Work out the finished part from the listing and answer in its coordinate system (mm). A direction names the side the tool comes from. Give positions to 0.01 mm unless a question says otherwise; leave off trailing zeros. Loops run counter-clockwise (first coordinate to the right, second up) from the corner with the lowest first, then second, coordinate; pieces in that order, holes last. Notation, with made-up numbers: (-36.75, 50) - (3.25, 50) arc R20 ccw to (3.25, 66) - close; hole circle Ø3 at (45, 31). An arc over 180 degrees is marked (long way). One line per item, written item: value.
Autodesk Inventor part; units mm, degrees
ref_plane "YZ Plane" through (0, 0, 0) normal (1, 0, 0) x (0, 1, 0)
ref_plane "XZ Plane" through (0, 0, 0) normal (0, 1, 0) x (-1, 0, 0)
ref_plane "XY Plane" through (0, 0, 0) normal (0, 0, 1) x (1, 0, 0)
sketch "Sketch1" plane through (0, 0, 0) normal (0, 1, 0) x (-1, 0, 0)
  line L0 (0, 0) -> (2.032, 0) construction
  line L1 (0, 0) -> (-2.032, 0) construction
  line L2 (-4.318, 0) -> (-4.318, 3.81)
  line L3 (-4.318, 3.81) -> (5.842, 3.81)
  line L4 (-2.032, 0) -> (-2.032, 1.651)
  line L5 (-2.032, 1.651) -> (2.032, 1.651)
  line L6 (2.032, -46.228) -> (-2.032, -46.228)
  line L7 (-2.032, -46.228) -> (-2.032, -44.577)
  line L8 (-4.318, -44.577) -> (-4.318, -48.387)
  line L9 (-4.318, -48.387) -> (5.842, -48.387)
  line L10 (2.032, 1.651) -> (2.032, -16.5735)
  line L11 (2.032, -16.5735) -> (4.572, -16.5735)
  line L12 (4.572, -16.5735) -> (4.572, -28.0035)
  line L13 (4.572, -28.0035) -> (2.032, -28.0035)
  line L14 (2.032, -28.0035) -> (2.032, -46.228)
  line L15 (5.842, 3.81) -> (5.842, -48.387)
  line L16 (-2.032, -40.8058) -> (4.191, -40.8058) construction
  line L17 (-2.032, 0) -> (-2.032, -44.577)
  line L18 (-4.318, 0) -> (-4.318, -44.577)
  dimension "d0" = 2.032
  dimension "d1" = 2.032
  dimension "d3" = 2.286
  dimension "d5" = 3.81
  dimension "d7" = 10.16
  dimension "d8" = 4.064
  dimension "d9" = 2.159
  dimension "d10" = 1.651
  dimension "d12" = 2.286
  dimension "d13" = 3.81
  dimension "d14" = 1.651
  dimension "d15" = 4.064
  dimension "d16" = 10.16
  dimension "d17" = 11.43
  dimension "d18" = 2.159
  dimension "d19" = 18.2245
  dimension "d21" = 6.223
  dimension "d22" = 2.54
  dimension "d37" = 18.2245
  dimension "d38" = 52.197
  dimension "d39" = 44.577
extrude "Extrusion1" add sketch "Sketch1" along normal blind 2.9845
sketch "Sketch10" plane through (0, 0, 0) normal (0, -1, 0) x (1, 0, 0)
  line L0 (-2.032, 1.651) -> (-2.032, -16.5735)
  line L1 (2.032, -46.228) -> (2.032, 1.651)
  line L2 (-2.032, 1.651) -> (2.032, 1.651)
  line L3 (2.032, 1.651) -> (2.032, -46.228)
  line L4 (2.032, -46.228) -> (-2.032, -46.228)
  line L5 (-2.032, -46.228) -> (-2.032, 1.651)
  point P0 (0, 0)
extrude "Extrusion5" add sketch "Sketch10" against normal blind 1.27
sketch "Sketch11" plane through (0, 2.9845, 0) normal (0, 1, 0) x (1, 0, 0)
  line L0 (4.318, -3.81) -> (-5.842, -3.81)
  line L1 (-5.842, -3.81) -> (-5.842, 48.387)
  line L2 (-5.842, -3.81) -> (-5.842, 48.387)
  line L3 (4.318, 48.387) -> (4.318, 44.577) construction
  line L4 (4.318, -3.81) -> (4.318, 48.387) construction
  line L5 (4.318, -3.81) -> (4.318, 0) construction
  line L6 (4.318, -3.81) -> (4.318, 0)
  line L7 (4.318, 0) -> (2.032, 0)
  line L8 (2.032, 46.228) -> (2.032, -1.651)
  line L9 (2.032, -1.651) -> (-2.032, -1.651)
  line L10 (2.032, -1.651) -> (-2.032, -1.651)
  line L11 (-2.032, 28.0035) -> (-2.032, 16.5735)
  line L12 (-2.032, -1.651) -> (-2.032, 16.5735)
  line L13 (-2.032, -1.651) -> (-2.032, 16.5735)
  line L14 (-4.572, 16.5735) -> (-2.032, 16.5735)
  line L15 (-2.032, 16.5735) -> (-4.572, 16.5735)
  line L16 (-4.572, 16.5735) -> (-4.572, 28.0035)
  line L17 (-4.572, 16.5735) -> (-4.572, 28.0035)
  line L18 (-2.032, 28.0035) -> (-4.572, 28.0035)
  line L19 (-4.572, 28.0035) -> (-2.032, 28.0035)
  line L20 (-2.032, 28.0035) -> (-2.032, 46.228)
  line L21 (-2.032, 46.228) -> (2.032, 46.228)
  line L22 (2.032, 46.228) -> (2.032, 44.577)
  line L23 (2.032, 44.577) -> (4.318, 44.577)
  line L24 (4.318, 44.577) -> (4.318, 48.387)
  line L25 (-5.842, 48.387) -> (4.318, 48.387)
  point P0 (0, 0)
  dimension "d43" = 3.81
  dimension "d44" = 3.81
extrude "Extrusion6" add sketch "Sketch11" along normal blind 20.701 contours L0 L1 L25 L24 L23 L8 L21 L20 L18 L16 L14 L12 L9 L7 L6
sketch "Sketch12" plane through (-5.842, 0, 3.81) normal (0, 0, 1) x (1, 0, 0)
  line L0 (0, 0) -> (0, 23.6855) construction
  line L1 (10.16, 0) -> (0, 0) construction
  line L2 (0, 0) -> (0, 23.6855)
  line L3 (0, 0) -> (-6.35, 0) construction
  line L4 (0, 0) -> (0, 6.35) construction
  arc A0 (0, 6.35) -> (-6.35, 0) centre (0, 0) ccw
  line L5 (-6.35, 0) -> (0, 0)
  line L6 (0, 0) -> (0, 6.35)
  point P0 (5.842, 0)
  dimension "d54" = 6.35
  dimension "d55" = 6.35
  dimension "d56" = 6.35
extrude "Extrusion7" add sketch "Sketch12" against normal blind 10.16
sketch "Sketch14" plane through (4.318, 0, -48.387) normal (0, 0, -1) x (-1, 0, 0)
  line L0 (10.16, 0) -> (0, 0)
  line L1 (10.16, 0) -> (10.16, 6.3521)
  line L2 (10.16, 0) -> (10.16, 23.6855)
  line L3 (0, 0) -> (16.51, 0)
  line L4 (10.16, 0) -> (16.51, 0)
  arc A0 (16.51, 0) -> (10.16, 6.3521) centre (10.1572, -0.0008) ccw
  point P0 (4.318, 0)
extrude "Extrusion8" add sketch "Sketch14" against normal blind 10.16
sketch "Sketch16" plane through (0, 0, 0) normal (0, -1, 0) x (1, 0, 0)
  line L0 (-12.192, -38.227) -> (-5.842, -38.227)
  line L1 (-5.842, -38.227) -> (-21.082, -38.227)
  line L2 (-21.082, -38.227) -> (-21.082, -6.35)
  line L3 (-21.082, -6.35) -> (-5.842, -6.35)
  line L4 (-5.842, -6.35) -> (-5.842, -38.227)
  point P0 (0, 0)
  point P1 (-12.192, -6.35)
  dimension "d63" = 15.24
extrude "Extrusion9" add sketch "Sketch16" against normal blind 3.81
sketch "Sketch17" plane through (0, 3.81, 0) normal (0, 1, 0) x (1, 0, 0)
  circle A0 centre (-13.462, 29.4323) radius 1.9844
  circle A1 centre (-13.2021, 15.1448) radius 1.9844
  line L0 (-5.842, 38.227) -> (-5.842, 6.35) construction
  line L1 (-5.842, 36.0862) -> (-21.082, 36.0862) construction
  line L2 (-21.082, 38.227) -> (-21.082, 6.35) construction
  line L3 (-21.082, 37.0641) -> (-13.462, 37.0641) construction
  line L4 (-10.9221, 38.227) -> (-21.082, 38.227) construction
  line L5 (-12.933, 38.227) -> (-12.933, 6.35) construction
  line L6 (-21.082, 6.35) -> (-12.192, 6.35) construction
  line L7 (-21.082, 6.35) -> (-10.922, 6.35) construction
  line L8 (-5.842, 6.35) -> (-10.922, 6.35) construction
  line L9 (-13.462, 29.4323) -> (-13.462, 38.227) construction
  line L10 (-13.2021, 15.1448) -> (-13.2021, 6.35) construction
  point P0 (0, 0)
  dimension "d66" = 3.9688
  dimension "d67" = 3.9688
  dimension "d68" = 15.24
  dimension "d69" = 7.62
  dimension "d70" = 31.877
  dimension "d72" = 7.62
  dimension "d90" = 14.2875
extrude "Extrusion10" cut sketch "Sketch17" against normal blind 3.81
sketch "Sketch18" plane through (4.318, 0, 3.81) normal (1, 0, 0) x (0, 0, -1)
  line L0 (0, 1.944) -> (52.197, 1.944) construction
  line L1 (52.197, 0) -> (52.197, 6.3521) construction
  line L2 (0, 0) -> (0, 23.6855) construction
  line L3 (0, 2.5647) -> (21.5265, 2.5647) construction
  line L4 (48.387, 2.9845) -> (3.81, 2.9845)
  line L5 (21.5265, 2.9845) -> (30.6705, 2.9845)
  line L6 (21.5265, 2.9845) -> (21.5265, 13.1445)
  line L7 (21.5265, 13.1445) -> (30.6705, 13.1445)
  line L8 (30.6705, 13.1445) -> (30.6705, 2.9845)
  point P0 (3.81, 0)
  dimension "d79" = 52.197
  dimension "d80" = 21.5265
  dimension "d82" = 10.16
extrude "Extrusion11" add sketch "Sketch18" against normal blind 2.286
sketch "Sketch20" plane through (0, 23.6855, 0) normal (0, 1, 0) x (1, 0, 0)
  line L0 (-4.572, 16.5735) -> (-4.572, 28.0035)
  line L1 (-4.572, 28.0035) -> (-5.0647, 28.0035)
  line L2 (-5.0647, 28.0035) -> (-5.0647, 16.5735)
  line L3 (-5.0647, 16.5735) -> (-4.572, 16.5735)
  line L4 (-4.572, 16.5735) -> (-4.572, 28.0035)
  point P0 (0, 0)
extrude "Extrusion12" cut sketch "Sketch20" against normal up to next
sketch "Sketch21" plane through (0, 1.27, 0) normal (0, 1, 0) x (1, 0, 0)
  line L0 (-2.032, 16.5735) -> (-1.2835, 16.5735)
  line L1 (-1.2835, 16.5735) -> (-1.2835, 27.9949)
  line L2 (-1.2835, 27.9949) -> (-2.032, 27.9949)
  line L3 (-2.032, 27.9949) -> (-2.032, 16.5735)
  point P0 (0, 0)
extrude "Extrusion13" cut sketch "Sketch21" against normal up to next
sketch "Sketch22" plane through (0, 0, 0) normal (0, -1, 0) x (1, 0, 0)
  line L0 (2.032, -26.8605) -> (4.318, -26.8605)
  line L1 (4.318, -26.8605) -> (4.318, -17.6876)
  line L2 (4.318, -48.387) -> (4.318, 3.81)
  line L3 (4.318, -26.8605) -> (6.858, -26.8605)
  line L4 (6.858, -26.8605) -> (6.858, -17.7165)
  line L5 (6.858, -17.7165) -> (4.318, -17.7165)
  line L6 (4.318, -17.7165) -> (4.318, -26.8605)
  point P0 (0, 0)
  dimension "d91" = 2.54
extrude "Extrusion14" add sketch "Sketch22" against normal up to surface (13.1445 mm away)
sketch "Sketch23" plane through (2.032, 13.1445, -17.7165) normal (0, 1, 0) x (1, 0, 0)
  line L0 (0, 9.144) -> (4.826, 9.144)
  line L1 (2.286, 0) -> (0, 0)
  line L2 (0, 9.144) -> (1.143, 9.144)
  line L3 (1.143, 9.144) -> (1.143, 0)
  line L4 (1.143, 0) -> (0, 0)
  line L5 (0, 0) -> (0, 9.144)
  point P0 (-2.032, -17.7165)
extrude "Extrusion15" cut sketch "Sketch23" against normal up to surface (10.16 mm away)
sketch "Sketch24" plane through (-5.842, 23.6855, 3.81) normal (0, 0, 1) x (1, 0, 0)
  line L0 (0, -17.3334) -> (0, 0)
  line L1 (-6.35, -23.6855) -> (-15.24, -23.6855)
  line L2 (-15.24, -23.6855) -> (0, -23.6855)
  line L3 (-15.24, -23.6855) -> (-15.24, -19.8755)
  line L4 (-15.24, -23.6855) -> (-15.24, -19.8755)
  line L5 (-5.0801, -19.8755) -> (0, -19.8755)
  line L6 (-15.24, -19.8755) -> (0, -19.8755)
  line L7 (0, -19.8755) -> (0, -23.6855)
  point P0 (5.842, -23.6855)
sketch "Sketch25" plane through (0, 3.81, 0) normal (0, 1, 0) x (1, 0, 0)
  line L0 (-15.4123, 29.8338) -> (-11.4776, 29.4323) construction
  circle A0 centre (-13.462, 29.4323) radius 1.9844 construction
  line L1 (-15.4464, 29.4323) -> (-11.4776, 29.4323) construction
  circle A1 centre (-13.462, 29.4323) radius 1.9844 construction
  point P0 (0, 0)
extrude "Extrusion16" add sketch "Sketch24" against normal up to surface (52.197 mm away)
sketch "Sketch26" plane through (0, 3.81, 0) normal (0, 1, 0) x (1, 0, 0)
  line L0 (-13.4927, 29.4297) -> (-13.4927, 21.7166) construction
  line L1 (6.858, 26.8605) -> (6.858, 17.7165) construction
  line L2 (6.858, 22.1055) -> (-21.082, 22.1055) construction
  line L3 (-21.082, -3.81) -> (-21.082, 48.387) construction
  line L4 (-13.4927, 0.6164) -> (-13.4927, 43.5947) construction
  line L5 (-11.4607, 0.6164) -> (-11.4607, 43.5947) construction
  line L6 (-15.5247, 43.5947) -> (-15.5247, 0.6164) construction
  arc A0 (-15.5247, 0.6164) -> (-11.4607, 0.6164) centre (-13.4927, 0.6164) ccw construction
  arc A1 (-11.4607, 43.5947) -> (-15.5247, 43.5947) centre (-13.4927, 43.5947) ccw construction
  line L7 (-13.4927, 0.6164) -> (-13.4927, 43.5947) construction
  line L8 (-11.4607, 0.6164) -> (-11.4607, 43.5947)
  line L9 (-15.5247, 43.5947) -> (-15.5247, 0.6164)
  arc A2 (-15.5247, 0.6164) -> (-11.4607, 0.6164) centre (-13.4927, 0.6164) ccw
  arc A3 (-11.4607, 43.5947) -> (-15.5247, 43.5947) centre (-13.4927, 43.5947) ccw
  point P0 (0, 0)
  point P1 (-13.4927, 22.1055)
  dimension "d98" = 4.064
extrude "Extrusion17" cut sketch "Sketch26" against normal up to next
fillet "Fillet1" radius 3.175 2 edges at (-21.082, 1.905, 3.81) (-21.082, 1.905, -48.387)
properties part number "better ultrasonic holder"
1. Flat-ended cylindrical pins translate along their axes: pin 1 Ø10 at (y, z) = (19, -37.5) entering from -X; pin 2 Ø1.1 at (x, z) = (3.5, -28.5) entering from +Y; pin 3 Ø4 at (x, z) = (-11, -27.5) entering from +Y. Find the tip coordinate at first contact, or state that the pin passes through.
Output:
pin 1: stops at x = -5.84
pin 2: stops at y = 2.98
pin 3: stops at y = 3.81
2. For faces 4 (the flat face through (4.318, 8, -45)), 5 (the cylindrical face through (-13.537, 1.932, 1.415)), 6 (the flat face through (-2.032, 12, -7)), 7 (the flat face through (5, 6, -17.716)), determine the directions among +Z, -Z, +X, -X, +Y, -Y from which every point of the face is accessible in a straight line to the end or side of a thin tool.
Output:
face 4: -Z, +X, +Y, -Y
face 5: +Y, -Y
face 6: +Y
face 7: +X, +Y
3. Section A-A (z = -34) is taken. Write down the section's boundary in (x, y).
Output:
outline: (-21.08, 0) - (-15.52, 0) - (-15.52, 3.81) - (-21.08, 3.81) - close; (-11.46, 0) - (4.32, 0) - (4.32, 2.98) - (2.03, 2.98) - (2.03, 1.27) - (-2.03, 1.27) - (-2.03, 23.69) - (-5.84, 23.69) - (-5.84, 3.81) - (-11.46, 3.81) - close
4. Section D-D (z = -43) is taken. Write down the section's boundary in (x, y), and give its area (3 significant figures).
Output:
outline: (-21.08, 0) - (-15.52, 0) - (-15.52, 3.81) - (-21.08, 3.81) - close; (-11.46, 0) - (4.32, 0) - (4.32, 2.98) - (2.03, 2.98) - (2.03, 1.27) - (-2.03, 1.27) - (-2.03, 23.69) - (-5.84, 23.69) - (-5.84, 6.35) arc R6.35 ccw to (-10.92, 3.81) - (-11.46, 3.81) - close
area: 154 mm²
5. Section C-C (y = 19.5) is taken. Write down the section's boundary in (x, z).
Output:
outline: (-5.84, -48.39) - (4.32, -48.39) - (4.32, -44.58) - (2.03, -44.58) - (2.03, -46.23) - (-2.03, -46.23) - (-2.03, -28) - (-5.06, -28) - (-5.06, -16.57) - (-2.03, -16.57) - (-2.03, 1.65) - (2.03, 1.65) - (2.03, 0) - (4.32, 0) - (4.32, 3.81) - (-5.84, 3.81) - close
6. The mould has two halves that part along Z. Classify faces 1 (the flat face through (0, 12, -46.228)), 2 (the flat face through (-7, 0, -22)), 3 (the flat face through (-2, 9, 3.81)): released by +Z, released by -Z, zero draft, split by the parting line, or undercut.
Output:
face 1: undercut
face 2: zero draft
face 3: released by +Z
7. Section B-B (y = 7.5) is taken. Write down the section's boundary in (x, z) (1 decimal), and give its area (3 significant figures).
Output:
outline: (-5.8, -48.4) - (4.3, -48.4) - (4.3, -44.6) - (2, -44.6) - (2, -46.2) - (-2, -46.2) - (-2, -28) - (-5.1, -28) - (-5.1, -16.6) - (-2, -16.6) - (-2, 1.7) - (2, 1.7) - (2, 0) - (4.3, 0) - (4.3, 3.8) - (-5.8, 3.8) - close; (3.2, -26.9) - (6.9, -26.9) - (6.9, -17.7) - (3.2, -17.7) - close
area: 233 mm²
8. Find the intervals of material crossed by line 1 along Z through (x, y) = (2.5, 9.25); line 2 along X through (y, z) = (2, -27); line 3 along X through (y, z) = (6.75, -2), in increasing order.
Output:
line 1: z = -48.39 to -44.58, 0 to 3.81
line 2: x = -21.08 to -15.52, -11.46 to -5.06, 2.03 to 4.32
line 3: x = -5.84 to -2.03
